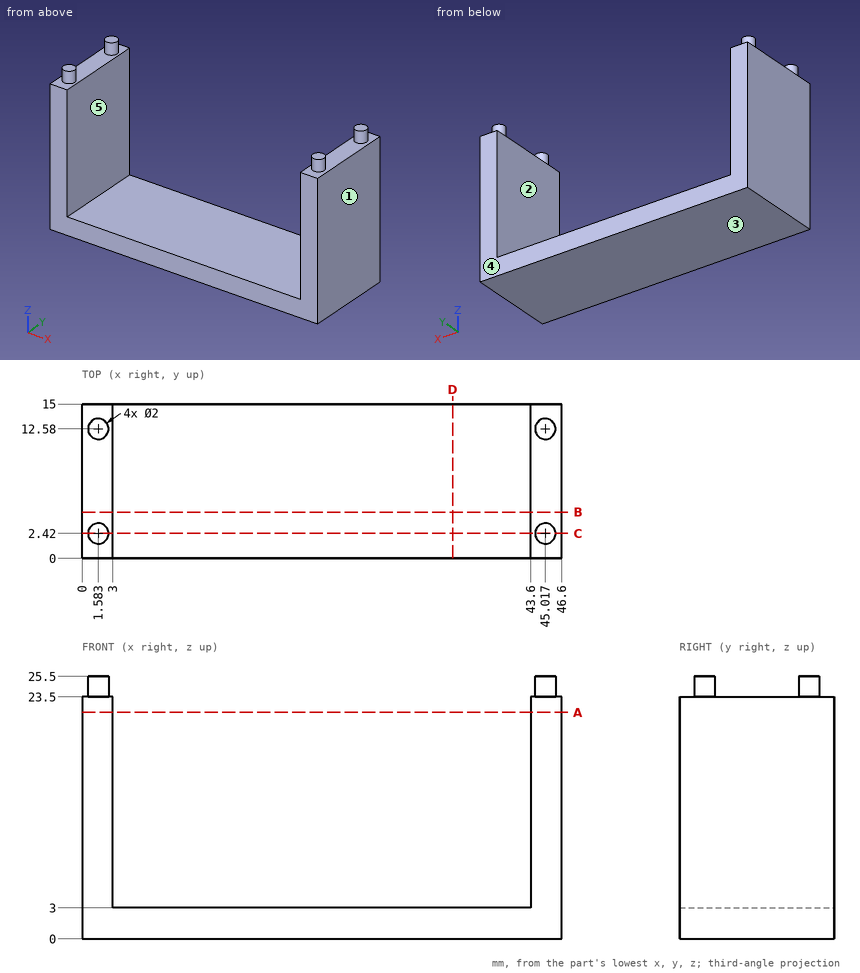
Geometry: see drawing. Coordinates: mm, zero at the bounding-box minimum. A direction names the side the tool comes from. Give positions to 0.01 mm unless a question says otherwise; leave off trailing zeros. Loops run counter-clockwise (first coordinate to the right, second up) from the corner with the lowest first, then second, coordinate; pieces in that order, holes last. Notation, with made-up numbers: (-37.75, 66) - (-26.75, 66) arc R9 ccw to (-26.75, 75) - close; hole circle Ø11 at (45, 81.25). An arc over 180 degrees is marked (long way). Use CSV: the item, a comma, the result in double quotes.
1) Set-up query: the marked faces 4 and 5. Return all of +Z, -Z, +X, -X, +Y, -Y with unobstructed straight access to the full face (end or side cutting, diameter ignored); none if empty.
Worked out:
face 4,"+Z, -Z, +X, -X, +Y"
face 5,"+Z, +Y, -Y"
2) Pin query (flat end, axial travel): P1, Ø0.9, axis at x = 1.5, y = 10, coming from the +Z side; P2, Ø2, axis at x = 8.5, y = 4, coming from the +Z side. Return the tip coordinate at first contact, or that it passes through.
Worked out:
P1,"stops at z = 23.5"
P2,"stops at z = 3"
3) Mould query, pull axis X, two halves, no side actions, for the marked faces 1, 2 and 3. Classes: +X half, -X half, draft (parallel to the pull), parting line (faces both ways), or undercut.
Worked out:
face 1,"+X half"
face 2,"undercut"
face 3,"draft"
4) Cut plane A-A (z = 22). Output: boundary loops of the cut face in (x, y).
Worked out:
outline,"(0, 0) - (3, 0) - (3, 15) - (0, 15) - close; (43.6, 0) - (46.6, 0) - (46.6, 15) - (43.6, 15) - close"
5) Cut plane D-D (x = 36). Output: boundary loops of the cut face in (y, z).
Worked out:
outline,"(0, 0) - (15, 0) - (15, 3) - (0, 3) - close"
6) Cut plane C-C (y = 2.42). Output: boundary loops of the cut face in (x, z).
Worked out:
outline,"(0, 0) - (46.6, 0) - (46.6, 23.5) - (46.02, 23.5) - (46.02, 25.5) - (44.02, 25.5) - (44.02, 23.5) - (43.6, 23.5) - (43.6, 3) - (3, 3) - (3, 23.5) - (2.58, 23.5) - (2.58, 25.5) - (0.58, 25.5) - (0.58, 23.5) - (0, 23.5) - close"
7) Cut plane B-B (y = 4.5). Output: boundary loops of the cut face in (x, z), and give its area (3 significant figures).
Worked out:
outline,"(0, 0) - (46.6, 0) - (46.6, 23.5) - (43.6, 23.5) - (43.6, 3) - (3, 3) - (3, 23.5) - (0, 23.5) - close"
area,"263 mm^2"
8) Line query: line 1 (X direction, y = 5.5, z = 13.5); line 2 (Z direction, x = 25, y = 5.5). Output: solid intervals per line, ascending.
Worked out:
line 1,"x = 0 to 3, 43.6 to 46.6"
line 2,"z = 0 to 3"
